Here's how the part is built. I have some questions about the finished solid (model axes, mm). A direction names the side the tool comes from. Coordinates: 2 decimals unless noted, no trailing zeros. Write each loop counter-clockwise with the first axis right and the second up, starting at its lowest first coordinate (ties: lowest second). Pieces come first, ordered by that corner, then holes.
Item 1: If we section it at C-C (y = -2.5): Please give me the cut outline in (x, z).
Item 2: If we section it at B-B (z = 0): Please give me the cut outline in (x, y), then the cut area to 3 significant figures.
Item 3: I'm going to push flat-ended pins straight in: pin 1 Ø4 at (x, y) = (19.5, -0.5) entering from +Z; pin 2 Ø1 at (x, y) = (-40.5, 4) entering from +Z; pin 3 Ø2 at (y, z) = (2.5, 39) entering from -X. Where does each tip first touch, or does it pass through?
Item 4: For faces 4 (the face through (5, 5, 51)), 5 (the face through (-37, 0, -37)), which set-ups out of +Z, -Z, +X, -X, +Y, -Y let a thin tool reach every point of the face, with its end or its side?
Item 5: We'd pull the mould along X, two halves only. Please class faces 1 (the face through (38, -5, -34)), 2 (the face through (-6.678, -2.465, -50.863)), 3 (the face through (-10.95, 0.07, 49.3)): +X half, -X half, draft (parallel to the pull), parting line (faces both ways), or undercut.
Item 6: If I drill on line 1 (X direction, y = 1, z = 0); line 2 (Z direction, x = 0, y = -2), over which ranges is the centre line in solid material (lowest first)?
Item 7: If we section it at A-A (x = 0): Please give me the cut outline in (y, z), then the cut area to 3 significant figures.
Autodesk Fusion 360 part; units mm, degrees
sketch "Sketch1" plane through (0, 0, 0) normal (0, 1, 0) x (1, 0, 0)
  circle A0 centre (0, 0) radius 50.5
  circle A1 centre (0, 0) radius 70
  dimension "d1" = 101
  dimension "d2" = 140
extrude "Extrude1" add sketch "Sketch1" along normal blind 5
chamfer "Chamfer1" distance 1 angle 45 1 edges at (-65.2629, 5, 25.3131)
sketch "Sketch2" plane through (0, 0, 0) normal (0, -1, 0) x (1, 0, 0)
  circle A0 centre (0, 0) radius 50.5
  circle A1 centre (0, 0) radius 70
  circle A2 centre (0, 0) radius 50.5
  circle A3 centre (0, 0) radius 51.3
  dimension "d6" = 102.6
extrude "Extrude2" add sketch "Sketch2" along normal blind 5 contours A3
equation "d6 = 101.000 mm + 0.8 * 2 mm"
Answer list:
1. outline: circle Ø102.6 at (0, 0); hole circle Ø101 at (0, 0)
2. outline: (-70, 0) - (-51.3, 0) - (-51.3, -5) - (-50.5, -5) - (-50.5, 5) - (-69, 5) - (-70, 4) - close; (50.5, -5) - (51.3, -5) - (51.3, 0) - (70, 0) - (70, 4) - (69, 5) - (50.5, 5) - close
2. area: 202 mm2
3. pin 1: stops at z = 67.76
3. pin 2: stops at z = 57.45
3. pin 3: stops at x = -58.79
4. face 4: +Z, -Z, +X, -X, +Y
4. face 5: -Y
5. face 1: draft
5. face 2: parting line
5. face 3: undercut
6. line 1: x = -70 to -50.5, 50.5 to 70
6. line 2: z = -51.3 to -50.5, 50.5 to 51.3
7. outline: (-5, -51.3) - (0, -51.3) - (0, -70) - (4, -70) - (5, -69) - (5, -50.5) - (-5, -50.5) - close; (-5, 50.5) - (5, 50.5) - (5, 69) - (4, 70) - (0, 70) - (0, 51.3) - (-5, 51.3) - close
7. area: 202 mm2
